Model file for the job. Use its own axes, mm. A direction names the side the tool comes from. Give positions to 0.01 mm unless a question says otherwise; leave off trailing zeros. Loops run counter-clockwise (first coordinate to the right, second up) from the corner with the lowest first, then second, coordinate; pieces in that order, holes last. Notation, with made-up numbers: (23.5, 59) - (61.5, 59) arc R17 cw to (61.5, 80) - close; hole circle Ø4 at (15.25, 7.5). An arc over 180 degrees is marked (long way). Use a Markdown table: item, result.
from build123d import *

# Parameters (mm, degrees)
F0_W     = 100
F0_H     = 15
F3_DEPTH = 55


with BuildPart() as f1:
    # F0 (on Front) → F1 (revolve)
    with BuildSketch(Plane.XZ):
        with Locations((0, 7.5)):
            Rectangle(F0_W, F0_H)
    revolve(axis=Axis((0, 0, 0), (1, 0, 0)))

    # F2 (on face) → F3 (cut)
    with BuildSketch(Plane(origin=(-50, 0, 0), x_dir=(0, -1, 0), z_dir=(-1, 0, 0))):
        with BuildLine():
            Line((3, 12), (3, 14.6969384567))
            ThreePointArc((3, 14.6969384567), (0, 15), (-3, 14.6969384567))
            Line((-3, 14.6969384567), (-3, 12))
            Line((-3, 12), (3, 12))
        make_face()
    extrude(amount=-F3_DEPTH, mode=Mode.SUBTRACT)


solid = f1.part
(1) Drill centre lines: probe 1 along X at (y, z) = (-0.5, 12.75); probe 2 along Y at (x, z) = (-43, 13.5); probe 3 along Y at (x, z) = (0, 0.25). Where is each one in solid material? Low to high. Write a range as [from, to].
Computed:
| item | result |
|---|---|
| probe 1 | [5, 50] |
| probe 2 | [-6.54, -3], [3, 6.54] |
| probe 3 | [-15, 15] |
(2) Pin check, flat tips, straight feed: P1, Ø5, axis at x = -10.5, z = 11, coming from the +Y side; P2, Ø1.3, axis at x = -14, z = 13, coming from the +Y side; P3, Ø10, axis at x = -30.5, y = 5.5, coming from the +Z side. Stop position of each tip, or through.
Computed:
| item | result |
|---|---|
| P1 | y = 12.36 |
| P2 | y = 8.51 |
| P3 | z = 14.7 |
(3) Slice it at A-A, the plane y = 0. Write the cut outline in (x, z), plus the area to 4 significant figures.
Computed:
| item | result |
|---|---|
| outline | (-50, -15) - (50, -15) - (50, 15) - (5, 15) - (5, 12) - (-50, 12) - close |
| area | 2,835 mm² |
(4) 3-axis set-ups, long thin cutter, end or side, ignore diameter. For faces 4 (the flat face through (-50, 0, 0)), 5 (the flat face through (5, 0, 14)): which of +Z, -Z, +X, -X, +Y, -Y reach the whole face in a straight line?
Computed:
| item | result |
|---|---|
| face 4 | +Z, -Z, -X, +Y, -Y |
| face 5 | +Z, -X |
(5) Slice it at D-D, the plane x = -22. Write the cut outline in (y, z).
Computed:
| item | result |
|---|---|
| outline | (-3, 12) - (-3, 14.7) arc R15 ccw (long way) to (3, 14.7) - (3, 12) - close |
(6) Slice it at C-C, the plane z = -5.5. Write the cut outline in (x, y), plus the area to 3 significant figures.
Computed:
| item | result |
|---|---|
| outline | (-50, -13.96) - (50, -13.96) - (50, 13.96) - (-50, 13.96) - close |
| area | 2,790 mm² |
(7) Slice it at B-B, the plane x = 7. Write the cut outline in (y, z), plus the area to 3 significant figures.
Computed:
| item | result |
|---|---|
| outline | circle Ø30 at (0, 0) |
| area | 707 mm² |
(8) Mould opens along Y. For faces 1 (the cylindrical face through (0.7, -4.506, 14.307)), 2 (the flat face through (-23, -3, 13)), 3 (the flat face through (50, 0, 0)) say: pulls with the +Y half, pulls with the -Y half, needs draft (parallel to the pull), parting line crosses it, or undercut.
Computed:
| item | result |
|---|---|
| face 1 | parting line crosses it |
| face 2 | undercut |
| face 3 | needs draft |
